from build123d import *

# Parameters (mm, degrees)
SALIENTE_EXTRUIR1_DEPTH = 2
SALIENTE_EXTRUIR2_DEPTH = 5
REDONDEO1_SIZE          = 2
CROQUIS3_W              = 30.87
CROQUIS3_H              = 2
CORTAR_EXTRUIR1_DEPTH   = 8


with BuildPart() as part:
    # Croquis1 → Saliente-Extruir1 (new body)
    with BuildSketch(Plane(origin=(0, 0, 0), x_dir=(1, 0, 0), z_dir=(0, 1, 0))):
        with BuildLine():
            Line((-40.87, -31.3), (40.87, -31.3))
            ThreePointArc((40.87, -31.3), (45.112640687, -29.542640687), (46.87, -25.3))
            Line((46.87, -25.3), (46.87, 25.3))
            ThreePointArc((46.87, 25.3), (45.112640687, 29.542640687), (40.87, 31.3))
            Line((40.87, 31.3), (-40.87, 31.3))
            ThreePointArc((-40.87, 31.3), (-45.112640687, 29.542640687), (-46.87, 25.3))
            Line((-46.87, 25.3), (-46.87, -25.3))
            ThreePointArc((-46.87, -25.3), (-45.112640687, -29.542640687), (-40.87, -31.3))
        make_face()
    extrude(amount=SALIENTE_EXTRUIR1_DEPTH)

    # Croquis2 → Saliente-Extruir2 (add)
    with BuildSketch(Plane(origin=(0, 2, 0), x_dir=(1, 0, 0), z_dir=(0, 1, 0))):
        with BuildLine():
            Line((44.87, -25.3), (44.87, 25.3))
            ThreePointArc((44.87, 25.3), (43.698427125, 28.128427125), (40.87, 29.3))
            Line((40.87, 29.3), (-40.87, 29.3))
            ThreePointArc((-40.87, 29.3), (-43.698427125, 28.128427125), (-44.87, 25.3))
            Line((-44.87, 25.3), (-44.87, -25.3))
            ThreePointArc((-44.87, -25.3), (-43.698427125, -28.128427125), (-40.87, -29.3))
            Line((-40.87, -29.3), (40.87, -29.3))
            ThreePointArc((40.87, -29.3), (43.698427125, -28.128427125), (44.87, -25.3))
        make_face()
        with BuildLine():
            Line((42.87, -25.3), (42.87, 25.3))
            ThreePointArc((42.87, 25.3), (42.284213562, 26.714213562), (40.87, 27.3))
            Line((40.87, 27.3), (-40.87, 27.3))
            ThreePointArc((-40.87, 27.3), (-42.284213562, 26.714213562), (-42.87, 25.3))
            Line((-42.87, 25.3), (-42.87, -25.3))
            ThreePointArc((-42.87, -25.3), (-42.284213562, -26.714213562), (-40.87, -27.3))
            Line((-40.87, -27.3), (40.87, -27.3))
            ThreePointArc((40.87, -27.3), (42.284213562, -26.714213562), (42.87, -25.3))
        make_face(mode=Mode.SUBTRACT)
    extrude(amount=SALIENTE_EXTRUIR2_DEPTH)

    # Redondeo1
    # a fillet whose section is not a circle: 2 mm, written as the material it takes off along each edge
    with BuildSketch(Plane(origin=(40.87, 7, -29.3), x_dir=(0, -1, 0), z_dir=(-1, 0, 0)), Plane(origin=(-40.87, 7, 29.3), x_dir=(0, -1, 0), z_dir=(1, 0, 0))) as redondeo1_piece_1:
        with BuildLine():
            Bezier((REDONDEO1_SIZE, 0), (0, 0), (0, REDONDEO1_SIZE), weights=[1, 0.111111111, 1])
            Line((0, REDONDEO1_SIZE), (0, 0))
            Line((0, 0), (REDONDEO1_SIZE, 0))
        make_face()
    extrude(amount=81.74, mode=Mode.SUBTRACT)
    with BuildSketch(Plane(origin=(-40.87, 7, -25.3), x_dir=(0, 0, -1), z_dir=(1, 0, 0))) as redondeo1_piece_2:
        with BuildLine():
            Bezier((4, -REDONDEO1_SIZE), (4, 0), (4 - REDONDEO1_SIZE, 0), weights=[1, 0.111111111, 1])
            Line((4 - REDONDEO1_SIZE, 0), (4, 0))
            Line((4, 0), (4, -REDONDEO1_SIZE))
        make_face()
    revolve(axis=Axis((-40.87, 7, -25.3), (0, 1, 0)), revolution_arc=90, mode=Mode.SUBTRACT)
    with BuildSketch(Plane(origin=(40.87, 7, -25.3), x_dir=(1, 0, 0), z_dir=(0, 0, 1))) as redondeo1_piece_3:
        with BuildLine():
            Bezier((4, -REDONDEO1_SIZE), (4, 0), (4 - REDONDEO1_SIZE, 0), weights=[1, 0.111111111, 1])
            Line((4 - REDONDEO1_SIZE, 0), (4, 0))
            Line((4, 0), (4, -REDONDEO1_SIZE))
        make_face()
    revolve(axis=Axis((40.87, 7, -25.3), (0, 1, 0)), revolution_arc=90, mode=Mode.SUBTRACT)
    with BuildSketch(Plane(origin=(-44.87, 7, -25.3), x_dir=(0, -1, 0), z_dir=(0, 0, 1)), Plane(origin=(44.87, 7, 25.3), x_dir=(0, -1, 0), z_dir=(0, 0, -1))) as redondeo1_piece_4:
        with BuildLine():
            Bezier((REDONDEO1_SIZE, 0), (0, 0), (0, REDONDEO1_SIZE), weights=[1, 0.111111111, 1])
            Line((0, REDONDEO1_SIZE), (0, 0))
            Line((0, 0), (REDONDEO1_SIZE, 0))
        make_face()
    extrude(amount=50.6, mode=Mode.SUBTRACT)
    with BuildSketch(Plane(origin=(-40.87, 7, 25.3), x_dir=(-1, 0, 0), z_dir=(0, 0, -1))) as redondeo1_piece_5:
        with BuildLine():
            Bezier((4, -REDONDEO1_SIZE), (4, 0), (4 - REDONDEO1_SIZE, 0), weights=[1, 0.111111111, 1])
            Line((4 - REDONDEO1_SIZE, 0), (4, 0))
            Line((4, 0), (4, -REDONDEO1_SIZE))
        make_face()
    revolve(axis=Axis((-40.87, 7, 25.3), (0, 1, 0)), revolution_arc=90, mode=Mode.SUBTRACT)
    with BuildSketch(Plane(origin=(40.87, 7, 25.3), x_dir=(0, 0, 1), z_dir=(-1, 0, 0))) as redondeo1_piece_6:
        with BuildLine():
            Bezier((4, -REDONDEO1_SIZE), (4, 0), (4 - REDONDEO1_SIZE, 0), weights=[1, 0.111111111, 1])
            Line((4 - REDONDEO1_SIZE, 0), (4, 0))
            Line((4, 0), (4, -REDONDEO1_SIZE))
        make_face()
    revolve(axis=Axis((40.87, 7, 25.3), (0, 1, 0)), revolution_arc=90, mode=Mode.SUBTRACT)

    # Croquis3 → Cortar-Extruir1 (cut)
    with BuildSketch(Plane(origin=(0, 2, 0), x_dir=(1, 0, 0), z_dir=(0, 1, 0))):
        with Locations((-20.435, -28.3)):
            Rectangle(CROQUIS3_W, CROQUIS3_H)
        with Locations((20.435, -28.3)):
            Rectangle(CROQUIS3_W, CROQUIS3_H)
    extrude(amount=CORTAR_EXTRUIR1_DEPTH, mode=Mode.SUBTRACT)


solid = part.part
Verification items for the finished model (mm, model axes). A direction names the side the tool comes from. Give positions to 0.01 mm unless a question says otherwise; leave off trailing zeros. Order: outer loops, then holes, each group sorted by start corner. A loop starts at its lowest first (then second) coordinate and runs counter-clockwise, first axis right, second up. Notation, with made-up numbers: M 82,83 L 92,83 A27 cw 92,113 Z; hole C 50,39.5 d1. An arc over 180 degrees is marked long. Use one line per item in the form item = value. Start each with the question number.
Q1. Scan lines: line 1 along X through (y, z) = (4.25, -7); line 2 along Z through (x, y) = (41, 2.25); line 3 along Z through (x, y) = (-14.5, 4). Record each from-to range of solid material in increasing order. Write a range as [from, to].
Q2. Section check A-A (y = 3). Enter the section's corners in (x, z).
Q3. Go/stop test with flat-tipped pins: pin 1 Ø1.6 at (y, z) = (5, 28.5) entering from +X; pin 2 Ø1.6 at (y, z) = (3.5, 28.5) entering from -X; pin 3 Ø1.5 at (x, y) = (-12.5, 5.5) entering from +Z. Record where each tip stops, or that it passes through.
Q4. Access from +Z, -Z, +X, -X, +Y, -Y to the whole of each face (thin tool, end or side, straight path). Record for faces 4 (the cylindrical face through (43.667, 3.479, 28.159)), 5 (the flat face through (-38, 3, 29.3)), 6 (the cylindrical face through (43.729, 3.479, -28.097)), 7 (the flat face through (-5, 4, 28)), 8 (the cylindrical face through (42.3, 4.5, -26.7)).
Q5. Mould release check, pull along X, two halves, no side actions. Record for faces 1 (the flat face through (-35.87, 4, 28)), 2 (the flat face through (44.87, 3, 0)), 3 (the flat face through (1, 3, -29.3)): +X half, -X half, draft (parallel to the pull), parting line (faces both ways), or undercut.
Evaluation:
q1.line_1 = [-44.87, -42.87], [42.87, 44.87]
q1.line_2 = [-29.3, -27.3], [27.3, 29.3]
q1.line_3 = [-29.3, -27.3]
q2.outline = M -44.87,-25.3 A4 ccw -40.87,-29.3 L 40.87,-29.3 A4 ccw 44.87,-25.3 L 44.87,25.3 A4 ccw 40.87,29.3 L 35.87,29.3 L 35.87,27.3 L 40.87,27.3 A2 cw 42.87,25.3 L 42.87,-25.3 A2 cw 40.87,-27.3 L -40.87,-27.3 A2 cw -42.87,-25.3 L -42.87,25.3 A2 cw -40.87,27.3 L -35.87,27.3 L -35.87,29.3 L -40.87,29.3 A4 ccw -44.87,25.3 Z; M -5,27.3 L 5,27.3 L 5,29.3 L -5,29.3 Z
q3.pin_1 = 44.07
q3.pin_2 = -44.07
q3.pin_3 = -27.3
q4.face_4 = +Z, +X, +Y
q4.face_5 = +Z, +X, -X, +Y
q4.face_6 = -Z, +X, +Y
q4.face_7 = +Z, +Y
q4.face_8 = +Y
q5.face_1 = undercut
q5.face_2 = +X half
q5.face_3 = draft
